Read the model definition and answer for the solid it produces. Units are mm, in the model's axes. Face numbers are marked on the shaded views. Coordinates: 2 decimals unless noted, no trailing zeros. Loops run counter-clockwise (first coordinate to the right, second up) from the corner with the lowest first, then second, coordinate; pieces in that order, holes last. Notation, with made-up numbers: M 21,-13.5 L 70,-13.5 A19 ccw 70,17.5 Z; hole C 19.5,87 d10. An arc over 180 degrees is marked long. Put each result on its own line as item: value.
from build123d import *

# Parameters (mm, degrees)
EXTRUDE1_DEPTH     = 12.446
SKETCH2_R          = 3.175
CUT_EXTRUDE1_DEPTH = 12.446


with BuildPart() as part:
    # Sketch1 → Extrude1 (new body)
    with BuildSketch(Plane.XY):
        with BuildLine():
            Line((-5.0927, 0), (5.0927, 0))
            ThreePointArc((5.0927, 0), (5.362107684, -0.111592316), (5.4737, -0.381))
            Line((5.4737, -0.381), (5.4737, -2.026133402))
            ThreePointArc((5.4737, -2.026133402), (5.448607976, -2.162113227), (5.37663694, -2.280182243))
            Line((5.37663694, -2.280182243), (3.644187879, -4.216448841))
            ThreePointArc((3.644187879, -4.216448841), (3.515763625, -4.3102172), (3.360250938, -4.3434))
            Line((3.360250938, -4.3434), (-3.360250938, -4.3434))
            ThreePointArc((-3.360250938, -4.3434), (-3.515763625, -4.3102172), (-3.644187879, -4.216448841))
            Line((-3.644187879, -4.216448841), (-5.37663694, -2.280182243))
            ThreePointArc((-5.37663694, -2.280182243), (-5.448607976, -2.162113227), (-5.4737, -2.026133402))
            Line((-5.4737, -2.026133402), (-5.4737, -0.381))
            ThreePointArc((-5.4737, -0.381), (-5.362107684, -0.111592316), (-5.0927, 0))
        make_face()
    extrude(amount=EXTRUDE1_DEPTH)

    # Sketch2 → Cut-Extrude1 (cut)
    with BuildSketch(Plane(origin=(0, 0, 0), x_dir=(-1, 0, 0), z_dir=(0, 1, 0))):
        with Locations((0, 5.08)):
            Circle(SKETCH2_R)
    extrude(amount=-CUT_EXTRUDE1_DEPTH, mode=Mode.SUBTRACT)


solid = part.part
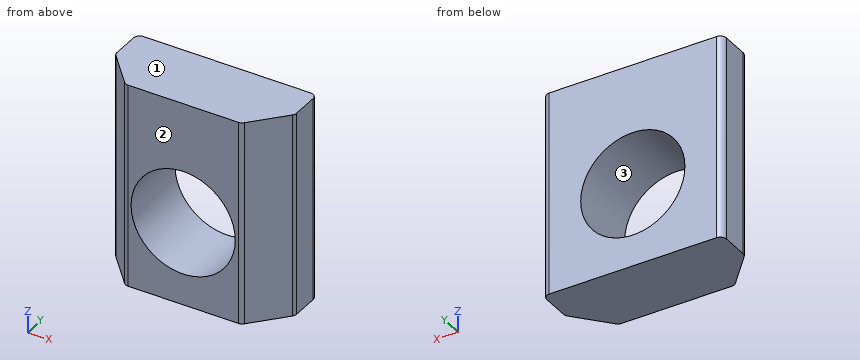
1) Find section A-A, the plane x = 0. Write down the section's boundary in (y, z) (3 decimals).
Answer list:
outline: M -4.343,0 L 0,0 L 0,1.905 L -4.343,1.905 Z; M -4.343,8.255 L 0,8.255 L 0,12.446 L -4.343,12.446 Z
2) Find section B-B, the plane z = 5.08. Write down the section's boundary in (x, y) (3 decimals), plus the area to 3 significant figures.
Answer list:
outline: M -5.474,-2.026 A0.381 ccw -5.377,-2.28 L -3.644,-4.216 A0.381 ccw -3.36,-4.343 L -3.175,-4.343 L -3.175,0 L -5.093,0 A0.381 ccw -5.474,-0.381 Z; M 3.175,-4.343 L 3.36,-4.343 A0.381 ccw 3.644,-4.216 L 5.377,-2.28 A0.381 ccw 5.474,-2.026 L 5.474,-0.381 A0.381 ccw 5.093,0 L 3.175,0 Z
area: 15.7 mm^2
3) Find section D-D, the plane z = 7.5. Write down the section's boundary in (x, y), plus the area to 3 significant figures.
Answer list:
outline: M -5.47,-2.03 A0.38 ccw -5.38,-2.28 L -3.64,-4.22 A0.38 ccw -3.36,-4.34 L -2.06,-4.34 L -2.06,0 L -5.09,0 A0.38 ccw -5.47,-0.38 Z; M 2.06,-4.34 L 3.36,-4.34 A0.38 ccw 3.64,-4.22 L 5.38,-2.28 A0.38 ccw 5.47,-2.03 L 5.47,-0.38 A0.38 ccw 5.09,0 L 2.06,0 Z
area: 25.4 mm^2
4) Find section C-C, the plane y = -1.4. Write down the section's boundary in (x, z) (3 decimals), plus the area to 3 significant figures.
Answer list:
outline: M -5.474,0 L 5.474,0 L 5.474,12.446 L -5.474,12.446 Z; hole C 0,5.08 d6.35
area: 105 mm^2
5) Straight lines are drawn through the part: line 1 (Z direction, x = 0, y = -1.1) (3 decimals); line 2 (X direction, y = -2.35, z = 7.5); line 3 (Z direction, x = -1.5, y = -3.4). For each, find the intervals that lie inside material, in ascending order. Write a range as [from, to].
Answer list:
line 1: z = [0, 1.905], [8.255, 12.446]
line 2: x = [-5.31, -2.06], [2.06, 5.31]
line 3: z = [0, 2.28], [7.88, 12.45]
6) Determine the mould class of the marked faces 1, 2 and 3 for opening direction Z: released by +Z, released by -Z, zero draft, split by the parting line, or undercut.
Answer list:
face 1: released by +Z
face 2: zero draft
face 3: undercut
